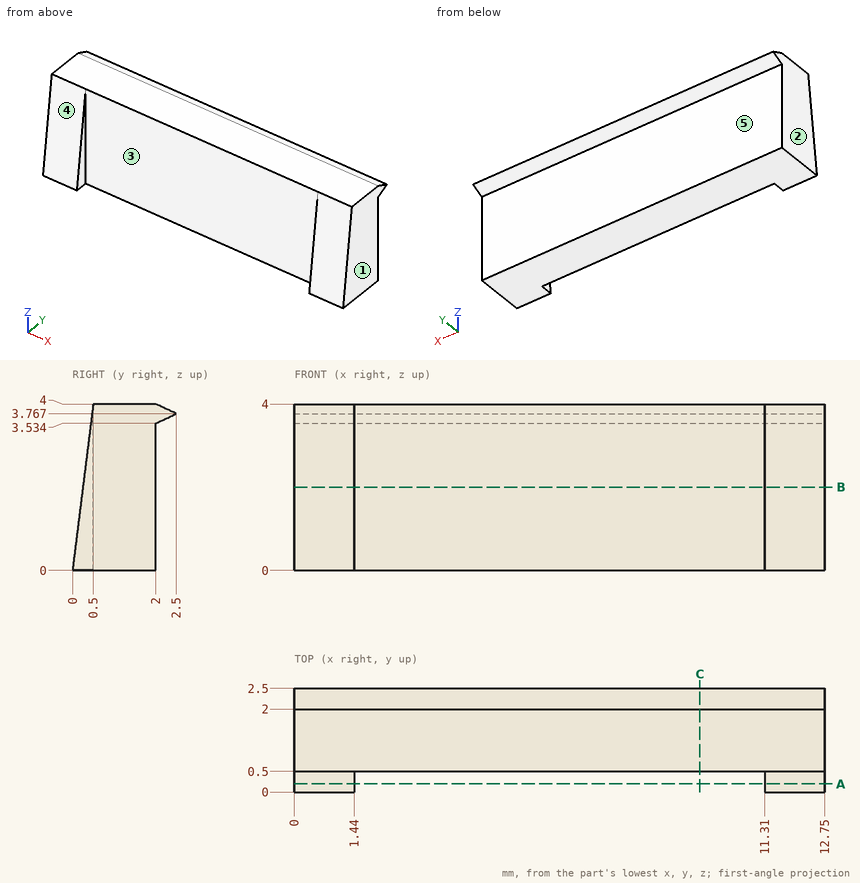
Geometry check sheet. Reference: drawing and pictorial views, mm from the part's lowest x, y, z. A direction names the side the tool comes from. Round coordinates to 2 decimals unless told otherwise and drop trailing zeros. Write each loop counter-clockwise with the first axis right and the second up, starting at its lowest first coordinate (ties: lowest second). Pieces come first, ordered by that corner, then holes. Notation, with made-up numbers: (-5.75, 13) -> (12.25, 13) arc R12 cw to (12.25, 23) -> close; hole circle Ø4 at (9, 9.5). An arc over 180 degrees is marked (long way). One line per question, with ' | ' between items. Start each with the question number.
1. Sectioned sample at A-A, the plane y = 0.2. Record the cut outline in (x, z).
2. Sectioned sample at B-B, the plane z = 2. Record the cut outline in (x, y).
3. Set-up check for the marked faces 4 and 5: record each of +Z, -Z, +X, -X, +Y, -Y from which the full face is reachable in a straight line by a thin tool's end or side.
4. Depth check by flat-ended pin: pin 1 (1.5 mm diameter, centred on x = 2.5, z = 2.5, fed in from -Y); pin 2 (1.8 mm diameter, centred on x = 9, z = 2, fed in from +Y). Enter the tip coordinate at first touch or a pass-through.
5. Scan lines: line 1 along Y through (x, z) = (5.5, 1.9); line 2 along Y through (x, z) = (3.75, 3.7) (1 decimal); line 3 along Z through (x, y) = (7.75, 2.05). Record each from-to range of solid material in increasing order. Write a range as from..to.
6. Sectioned sample at C-C, the plane x = 9.75. Record the cut outline in (y, z).
7. Release check for a two-part mould opening along X. For the marked faces 1, 2 and 3 record: +X half, -X half, draft (parallel to the pull), parting line (faces both ways), or undercut.
Taken from the geometry:
1) outline: (0, 0) -> (1.44, 0) -> (1.44, 1.6) -> (0, 1.6) -> close; (11.31, 0) -> (12.75, 0) -> (12.75, 1.6) -> (11.31, 1.6) -> close
2) outline: (0, 0.25) -> (1.44, 0.25) -> (1.44, 0.5) -> (11.31, 0.5) -> (11.31, 0.25) -> (12.75, 0.25) -> (12.75, 2) -> (0, 2) -> close
3) face 4: +Z, +X, -X, -Y | face 5: -Z, +X, -X, +Y
4) pin 1: stops at y = 0.5 | pin 2: stops at y = 2
5) line 1: y = 0.5..2 | line 2: y = 0.5..2.4 | line 3: z = 3.56..3.98
6) outline: (0.5, 0) -> (2, 0) -> (2, 3.53) -> (2.5, 3.77) -> (2, 4) -> (0.5, 4) -> close
7) face 1: +X half | face 2: -X half | face 3: undercut
